For this review, use the dimensioned drawing (mm, ordinates from the lowest corner) and the shaded views. Coordinates: 2 decimals unless noted, no trailing zeros. Loops run counter-clockwise (first coordinate to the right, second up) from the corner with the lowest first, then second, coordinate; pieces in that order, holes last. Notation, with made-up numbers: (-14, -9) - (-2, -9) arc R26 ccw to (-2, 25) - close; hole circle Ø3 at (24.25, -39.5). An arc over 180 degrees is marked (long way). Use one line per item in the form item = value. Start each with the question number.
(1) For L1, parallel to Y at x = 95, z = 2; L2, parallel to X at y = 19, z = 3.75, list the stretches that pass through material, from the lowest coordinate up.
(2) Add section B-B (y = 23). State the section outline as (x, z) points.
(3) Clearance check with flat-ended pins moving along their axes: pin 1 Ø1 at (x, z) = (110.5, 5) entering from +Y; pin 2 Ø5 at (y, z) = (77.5, 3) entering from +X; pin 3 Ø3 at (y, z) = (64.5, 3) entering from -X. State where each tip first meets the part, or that it passes through.
(4) Add section A-A (x = 25.5). State the section outline as (y, z) points, plus the area to 3 significant figures.
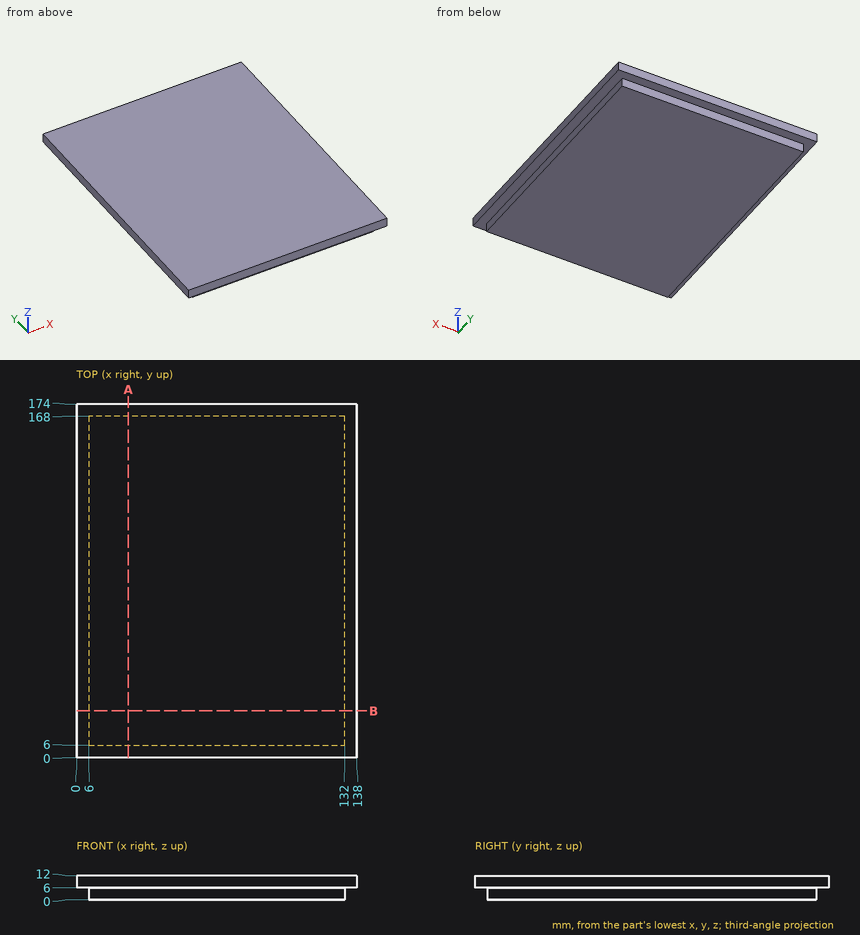
Computed values:
q1.L1 = 6 to 168
q1.L2 = 6 to 132
q2.outline = (0, 6) - (6, 6) - (6, 0) - (132, 0) - (132, 6) - (138, 6) - (138, 12) - (0, 12) - close
q3.pin_1 = 168
q3.pin_2 = 132
q3.pin_3 = 6
q4.outline = (0, 6) - (6, 6) - (6, 0) - (168, 0) - (168, 6) - (174, 6) - (174, 12) - (0, 12) - close
q4.area = 2,020 mm^2
